Answer from the drawing. Dimensions are ordinates in mm from the lowest x, y and z of the part. Round coordinates to 2 decimals unless told otherwise and drop trailing zeros. Write each loop counter-clockwise with the first axis right and the second up, starting at its lowest first coordinate (ties: lowest second). Pieces come first, ordered by that corner, then holes. Notation, with made-up numbers: M 85.5,53.5 L 131.5,53.5 A27 cw 131.5,90.5 Z; hole C -26.5,79 d11. An arc over 180 degrees is marked long. One line per item, written item: value. Start each with the question number.
(1) Given P1, Ø3, axis at x = 90.5, y = 76.5, coming from the +Z side, flat-ended and moving along its own axis, determine where the tip first touches the part or whether it passes through.
(2) For a pull along Y with two mould halves and no side action, classify the marked faces 1 and 2 as released by +Y, released by -Y, zero draft, split by the parting line, or undercut.
(3) Section B-B (y = 30) is taken. Determine the outline of the cut face in (x, z), plus the area to 3 significant figures.
(4) Section A-A (z = 10) is taken. Determine the outline of the cut face in (x, y), plus the area to 3 significant figures.
(5) Consider probe 1 along Y at (x, z) = (38, 6.25); probe 2 along X at (y, z) = (40.5, 10.5); probe 3 along Z at (x, y) = (162.5, 52). Determine where each line is inside the solid, lowest interval first.
(6) Section C-C (x = 54.5) is taken. Determine the outline of the cut face in (y, z).
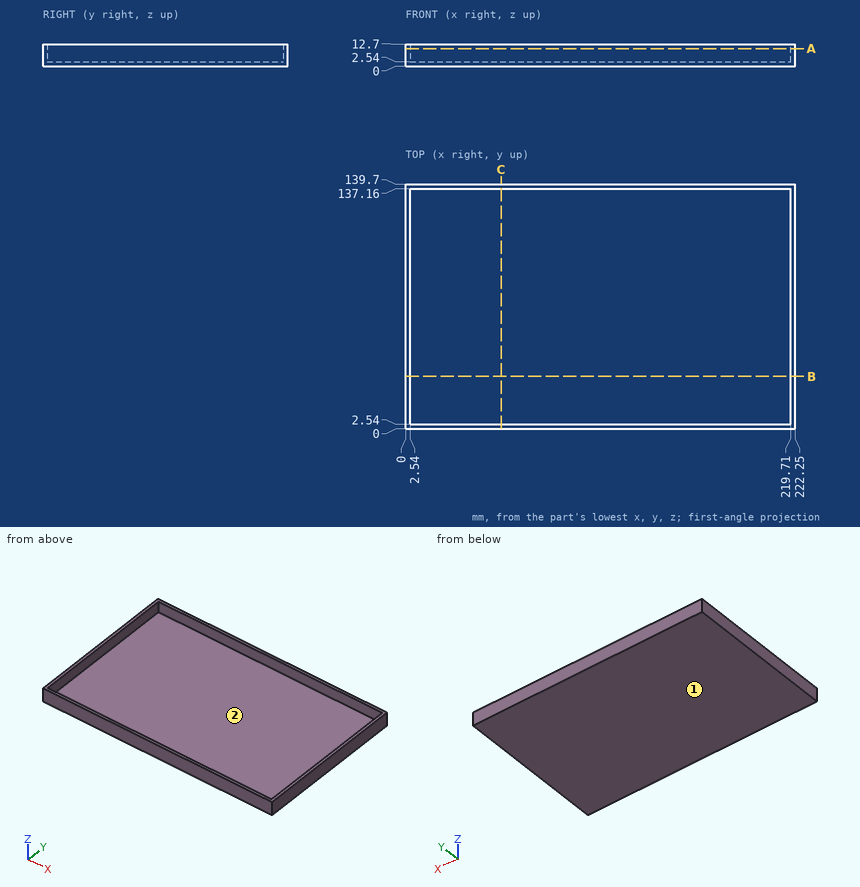
Recorded:
1. P1: stops at z = 2.54
2. face 1: zero draft
2. face 2: undercut
3. outline: M 0,0 L 222.25,0 L 222.25,12.7 L 219.71,12.7 L 219.71,2.54 L 2.54,2.54 L 2.54,12.7 L 0,12.7 Z
3. area: 616 mm2
4. outline: M 0,0 L 222.25,0 L 222.25,139.7 L 0,139.7 Z; hole M 2.54,2.54 L 219.71,2.54 L 219.71,137.16 L 2.54,137.16 Z
4. area: 1,810 mm2
5. probe 1: y = 0 to 2.54, 137.16 to 139.7
5. probe 2: x = 0 to 2.54, 219.71 to 222.25
5. probe 3: z = 0 to 2.54
6. outline: M 0,0 L 139.7,0 L 139.7,12.7 L 137.16,12.7 L 137.16,2.54 L 2.54,2.54 L 2.54,12.7 L 0,12.7 Z
